Verification items for the finished model (mm, model axes). A direction names the side the tool comes from. Coordinates: 2 decimals unless noted, no trailing zeros. Order: outer loops, then holes, each group sorted by start corner. A loop starts at its lowest first (then second) coordinate and runs counter-clockwise, first axis right, second up. Notation, with made-up numbers: (-26, 28.25) - (-4, 28.25) arc R16 cw to (-4, 33.25) - close; hole circle Ø8 at (-10.5, 63). An arc over 180 degrees is marked (long way). Answer as CSV lines item,"result". Start each with the question number.
1. Go/stop test with flat-tipped pins: pin 1 (2.5 mm diameter, centred on y = -5.5, z = 6, fed in from +X); pin 2 (2.5 mm diameter, centred on y = 6, z = 6, fed in from +X); pin 3 (0.6 mm diameter, centred on x = 1, z = 2, fed in from -Y). Record where each tip stops, or that it passes through.
2. Section check C-C (z = 7.25). Record the cut outline in (x, y), and give its area (3 significant figures).
3. Material ranges on L1, parallel to Z at x = -1.25, y = 2.5; L2, parallel to Y at x = 0.5, z = 2.75; L3, parallel to X at y = -3, z = 4.75 (3 decimals), recorded low to high. Write a range as [from, to].
4. Section check A-A (z = 3). Record the cut outline in (x, y), and give its area (3 significant figures).
5. Section check D-D (y = 2.5). Record the cut outline in (x, z), and give its area (3 significant figures).
6. Section check B-B (x = -2.25). Record the cut outline in (y, z).
7. Mould release check, pull along X, two halves, no side actions. Record for faces 1 (the flat face through (-2, 0, 6)), 2 (the flat face through (-1, 0, 4)), 3 (the flat face through (4.726, 2.871, 3.944)), 4 (the flat face through (3, 1.35, 4)): pulls with the +X half, pulls with the -X half, needs draft (parallel to the pull), parting line crosses it, or undercut.
8. Set-up check for faces 5 (the flat face through (1, -4.05, 4)), 6 (the flat face through (3, -1.35, 4)), 7 (the flat face through (-2, 0, 2)): record each of +Z, -Z, +X, -X, +Y, -Y from which the full face is reachable in a straight line by a thin tool's end or side.
from build123d import *

# Parameters (mm, degrees)
PAD_DEPTH       = 8
SKETCH001_W     = 6
SKETCH001_H     = 15
PAD001_DEPTH    = 8
SKETCH002_R     = 34.097943
POCKET_DEPTH    = 8.001
SKETCH003_W     = 2
SKETCH003_H     = 4
POCKET001_DEPTH = 15.001
POCKET002_DEPTH = 8.001


with BuildPart() as part:
    # Sketch → Pad (new body)
    with BuildSketch(Plane.XY):
        Polygon((6.5, 1.35), (0, 1.35), (0, -1.35), (6.5, -1.35), (3, -4.35), (0, -4.05), (-6, -4.05), (-6, 4.05), (0, 4.05), (3, 4.35), align=None)
    extrude(amount=PAD_DEPTH)

    # Sketch001 (on Face12 of Pad) → Pad001 (join)
    with BuildSketch(Plane.XY.offset(8)):
        with Locations((-3, 0)):
            Rectangle(SKETCH001_W, SKETCH001_H)
    extrude(amount=-PAD001_DEPTH)

    # Sketch002 (on Face13 of Pad001) → Pocket (cut, through all)
    with BuildSketch(Plane.XY.offset(8)):
        with Locations((-39.312778, 0)):
            Circle(SKETCH002_R)
    extrude(amount=-POCKET_DEPTH, mode=Mode.SUBTRACT)

    # Sketch003 (on Face15 of Pocket) → Pocket001 (cut, through all)
    with BuildSketch(Plane(origin=(0, 7.5, 0), x_dir=(-1, 0, 0), z_dir=(0, 1, 0))):
        with Locations((2, 4)):
            Rectangle(SKETCH003_W, SKETCH003_H)
    extrude(amount=-POCKET001_DEPTH, mode=Mode.SUBTRACT)

    # Sketch004 (on Face3 of Pocket001) → Pocket002 (cut, through all)
    with BuildSketch(Plane.XY.offset(8)):
        with BuildLine():
            ThreePointArc((0, 4.55), (-0.25, 4.3), (0, 4.05))
            Line((0, 4.05), (2.1, 4.05))
            ThreePointArc((2.1, 4.05), (2.35, 4.3), (2.1, 4.55))
            Line((0, 4.55), (2.1, 4.55))
        make_face()
        with BuildLine():
            ThreePointArc((0, -4.05), (-0.25, -4.3), (0, -4.55))
            Line((0, -4.55), (2.1, -4.55))
            ThreePointArc((2.1, -4.55), (2.35, -4.3), (2.1, -4.05))
            Line((0, -4.05), (2.1, -4.05))
        make_face()
    extrude(amount=-POCKET002_DEPTH, mode=Mode.SUBTRACT)


solid = part.part
Evaluation:
1,pin 1,"stops at x = 3.12"
1,pin 2,"stops at x = 0"
1,pin 3,"stops at y = -4.05"
2,outline,"(-6, -7.5) - (0, -7.5) - (0, -4.55) arc R0.25 cw to (0, -4.05) - (2.1, -4.05) arc R0.25 cw to (2.35, -4.28) - (3, -4.35) - (6.5, -1.35) - (0, -1.35) - (0, 1.35) - (6.5, 1.35) - (3, 4.35) - (2.35, 4.28) arc R0.25 cw to (2.1, 4.05) - (0, 4.05) arc R0.25 cw to (0, 4.55) - (0, 7.5) - (-6, 7.5) - (-6, 7.28) arc R34.1 cw to (-6, -7.28) - close"
2,area,"109 mm²"
3,L1,"z = [0, 2], [6, 8]"
3,L2,"y = [-4.05, -1.35], [1.35, 4.05]"
3,L3,"x = [-5.347, -3], [-1, 4.575]"
4,outline,"(-6, -7.5) - (-3, -7.5) - (-3, 7.5) - (-6, 7.5) - (-6, 7.28) arc R34.1 cw to (-6, -7.28) - close; (-1, -7.5) - (0, -7.5) - (0, -4.55) arc R0.25 cw to (0, -4.05) - (2.1, -4.05) arc R0.25 cw to (2.35, -4.28) - (3, -4.35) - (6.5, -1.35) - (0, -1.35) - (0, 1.35) - (6.5, 1.35) - (3, 4.35) - (2.35, 4.28) arc R0.25 cw to (2.1, 4.05) - (0, 4.05) arc R0.25 cw to (0, 4.55) - (0, 7.5) - (-1, 7.5) - close"
4,area,"79.2 mm²"
5,outline,"(-5.31, 0) - (5.16, 0) - (5.16, 8) - (-5.31, 8) - close; hole (-3, 2) - (-1, 2) - (-1, 6) - (-3, 6) - close"
5,area,"75.7 mm²"
6,outline,"(-7.5, 0) - (7.5, 0) - (7.5, 2) - (-7.5, 2) - close; (-7.5, 6) - (7.5, 6) - (7.5, 8) - (-7.5, 8) - close"
7,face 1,"undercut"
7,face 2,"undercut"
7,face 3,"pulls with the +X half"
7,face 4,"needs draft"
8,face 5,"+Z, -Z, -Y"
8,face 6,"+Z, -Z, +X"
8,face 7,"+Y, -Y"
